from build123d import *

# Parameters (mm, degrees)
SKETCH1_W           = 16
SKETCH1_H           = 4
BOSS_EXTRUDE1_DEPTH = 1.5
SKETCH2_W           = 0.5
SKETCH2_H           = 0.5
CUT_EXTRUDE1_DEPTH  = 2
SKETCH3_R           = 0.6
BOSS_EXTRUDE2_DEPTH = 2.5
BOSS_EXTRUDE2_TAPER = 1


with BuildPart() as part:
    # Sketch1 → Boss-Extrude1 (new body)
    with BuildSketch(Plane(origin=(0, 0, 0), x_dir=(1, 0, 0), z_dir=(0, 1, 0))):
        with Locations((8, 2)):
            Rectangle(SKETCH1_W, SKETCH1_H)
    extrude(amount=BOSS_EXTRUDE1_DEPTH)

    # Sketch2 → Cut-Extrude1 (cut)
    with BuildSketch(Plane(origin=(0, 1.5, 0), x_dir=(1, 0, 0), z_dir=(0, 1, 0))):
        with Locations((3, 3)):
            Rectangle(SKETCH2_W, SKETCH2_H)
        with Locations((1, 3)):
            Rectangle(SKETCH2_W, SKETCH2_H)
        with Locations((5, 3)):
            Rectangle(SKETCH2_W, SKETCH2_H)
        with Locations((7, 3)):
            Rectangle(SKETCH2_W, SKETCH2_H)
        with Locations((9, 3)):
            Rectangle(SKETCH2_W, SKETCH2_H)
        with Locations((11, 3)):
            Rectangle(SKETCH2_W, SKETCH2_H)
        with Locations((13, 3)):
            Rectangle(SKETCH2_W, SKETCH2_H)
        with Locations((15, 3)):
            Rectangle(SKETCH2_W, SKETCH2_H)
        with Locations((17, 3)):
            Rectangle(SKETCH2_W, SKETCH2_H)
        with Locations((19, 3)):
            Rectangle(SKETCH2_W, SKETCH2_H)
        with Locations((21, 3)):
            Rectangle(SKETCH2_W, SKETCH2_H)
        with Locations((23, 3)):
            Rectangle(SKETCH2_W, SKETCH2_H)
        with Locations((25, 3)):
            Rectangle(SKETCH2_W, SKETCH2_H)
        with Locations((27, 3)):
            Rectangle(SKETCH2_W, SKETCH2_H)
        with Locations((29, 3)):
            Rectangle(SKETCH2_W, SKETCH2_H)
        with Locations((31, 3)):
            Rectangle(SKETCH2_W, SKETCH2_H)
        with Locations((33, 3)):
            Rectangle(SKETCH2_W, SKETCH2_H)
        with Locations((35, 3)):
            Rectangle(SKETCH2_W, SKETCH2_H)
        with Locations((1, 1)):
            Rectangle(SKETCH2_W, SKETCH2_H)
        with Locations((3, 1)):
            Rectangle(SKETCH2_W, SKETCH2_H)
        with Locations((5, 1)):
            Rectangle(SKETCH2_W, SKETCH2_H)
        with Locations((7, 1)):
            Rectangle(SKETCH2_W, SKETCH2_H)
        with Locations((9, 1)):
            Rectangle(SKETCH2_W, SKETCH2_H)
        with Locations((11, 1)):
            Rectangle(SKETCH2_W, SKETCH2_H)
        with Locations((13, 1)):
            Rectangle(SKETCH2_W, SKETCH2_H)
        with Locations((15, 1)):
            Rectangle(SKETCH2_W, SKETCH2_H)
        with Locations((17, 1)):
            Rectangle(SKETCH2_W, SKETCH2_H)
        with Locations((19, 1)):
            Rectangle(SKETCH2_W, SKETCH2_H)
        with Locations((21, 1)):
            Rectangle(SKETCH2_W, SKETCH2_H)
        with Locations((23, 1)):
            Rectangle(SKETCH2_W, SKETCH2_H)
        with Locations((25, 1)):
            Rectangle(SKETCH2_W, SKETCH2_H)
        with Locations((27, 1)):
            Rectangle(SKETCH2_W, SKETCH2_H)
        with Locations((29, 1)):
            Rectangle(SKETCH2_W, SKETCH2_H)
        with Locations((31, 1)):
            Rectangle(SKETCH2_W, SKETCH2_H)
        with Locations((33, 1)):
            Rectangle(SKETCH2_W, SKETCH2_H)
        with Locations((35, 1)):
            Rectangle(SKETCH2_W, SKETCH2_H)
    extrude(amount=-CUT_EXTRUDE1_DEPTH, mode=Mode.SUBTRACT)

    # Sketch3 → Boss-Extrude2 (add)
    with BuildSketch(Plane(origin=(0, 0, 0), x_dir=(1, 0, 0), z_dir=(0, 1, 0))):
        with Locations((2, 2)):
            Circle(SKETCH3_R)
        with Locations((14, 2)):
            Circle(SKETCH3_R)
    extrude(amount=-BOSS_EXTRUDE2_DEPTH, taper=BOSS_EXTRUDE2_TAPER)


solid = part.part
Can you work these out from the model? Positions are in its coordinate system, mm. A direction names the side the tool comes from. Give positions to 0.01 mm unless a question says otherwise; leave off trailing zeros. Order: outer loops, then holes, each group sorted by start corner. A loop starts at its lowest first (then second) coordinate and runs counter-clockwise, first axis right, second up. Notation, with made-up numbers: M 67.25,10 L 108.25,10 A29 cw 108.25,36 Z; hole C 45.25,32 d11. An arc over 180 degrees is marked long. Use a Markdown table: item, result. Add a question column.
Item 1: We'd pull the mould along X, two halves only. Please class faces 3 (the flat face through (0, 1, -2)), 4 (the flat face through (8, 0, -2)), 5 (the flat face through (8, 1, -4)), 6 (the conical face through (2.551, -1.268, -2.174)): +X half, -X half, draft (parallel to the pull), parting line (faces both ways), or undercut.
Item 2: Suppose I cut it at C-C (x = 8). List the corners of the cut face in (y, z) for me, then the cut area to 3 significant figures.
Item 3: Suppose I cut it at A-A (z = -1.05). Count the separate pieces of the cut face and the enclosed holes in it, then the cut area to 3 significant figures.
Item 4: Will this pin go through, and if not, where does the flat tip stop? pin 1 (1.5 mm diameter, centred on x = 4, y = -1, fed in from -Z).
Item 5: For faces 1 (the flat face through (8, 1.5, -2)), 2 (the conical face through (13.54, -1.27, -1.65)), which set-ups out of +Z, -Z, +X, -X, +Y, -Y let a thin tool reach every point of the face, with its end or its side?
Item 6: Suppose I cut it at B-B (y = -0.5). List the corners of the cut face in (x, z) for me.
Item 7: If I drill on L1, parallel to Y at x = 15.25, z = -1.45; L2, parallel to X at y = -1.4, z = -2.25; L3, parallel to X at y = -1.5, z = -2.5, over which ranges is the centre line in solid material (lowest first)? Write a range as [from, to].
Answer sheet:
| question | item | result |
|---|---|---|
| 1 | face 3 | -X half |
| 1 | face 4 | undercut |
| 1 | face 5 | draft |
| 1 | face 6 | undercut |
| 2 | outline | M 0,-4 L 1.5,-4 L 1.5,0 L 0,0 Z |
| 2 | area | 6.00 mm² |
| 3 | separate pieces | 9 |
| 3 | enclosed holes | 0 |
| 3 | area | 18.0 mm² |
| 4 | pin 1 | passes through |
| 5 | face 1 | +Z, -Z, +X, -X, +Y |
| 5 | face 2 | -Y |
| 6 | outline | C 2,-2 d1.18; C 14,-2 d1.18 |
| 7 | L1 | y = [0, 1.5] |
| 7 | L2 | x = [1.48, 2.52], [13.48, 14.52] |
| 7 | L3 | x = [1.72, 2.28], [13.72, 14.28] |
